Read the model definition and answer for the solid it produces. Units are mm, in the model's axes. Coordinates: 2 decimals unless noted, no trailing zeros. Loops run counter-clockwise (first coordinate to the right, second up) from the corner with the lowest first, then second, coordinate; pieces in that order, holes last.
Q1. Section B-B (y = 22.5) is taken. Give the vertices of the cut face in (x, z).
Q2. Flat-ended cylindrical pins translate along their axes: P1, Ø1.5, axis at x = 2, z = -83, coming from the -Y side; P2, Ø1.5, axis at x = 1.5, z = -104.5, coming from the -Y side. Find the tip coordinate at first contact, or state that the pin passes through.
Q3. Straight lines are drawn through the part: line 1 (Z direction, x = 0.4, y = 9); line 2 (Y direction, x = 2.55, z = -91). For each, find the intervals that lie inside material, in ascending order.
Q4. Section A-A (x = 0.5) is taken. Give the vertices of the cut face in (y, z).
Autodesk Inventor part; units mm, degrees
ref_plane "YZ Plane" through (0, 0, 0) normal (1, 0, 0) x (0, 1, 0)
ref_plane "XZ Plane" through (0, 0, 0) normal (0, 1, 0) x (-1, 0, 0)
ref_plane "XY Plane" through (0, 0, 0) normal (0, 0, 1) x (1, 0, 0)
sketch "Boceto1" plane through (0, 0, 0) normal (1, 0, 0) x (0, 1, 0)
  line L0 (0, 0) -> (24.8, 0)
  line L1 (24.8, 0) -> (24.8, -89.7)
  line L2 (24.8, -89.7) -> (0, -89.7)
  line L3 (0, -89.7) -> (0, 0)
  line L4 (0, -44.85) -> (73, -44.85) construction
  line L5 (24.8, -44.85) -> (73, -44.85) construction
  line L6 (24.8, 25.15) -> (73, 25.15)
  line L7 (73, 25.15) -> (73, -114.85)
  line L8 (73, -114.85) -> (24.8, -114.85)
  line L9 (24.8, -114.85) -> (24.8, 25.15)
  line L10 (24.8, 25.15) -> (73, -114.85) construction
  line L11 (73, 25.15) -> (24.8, -114.85) construction
  point P0 (48.9, -44.85)
  dimension "d0" = 24.8
  dimension "d1" = 89.7
  dimension "d2" = 73
  dimension "d3" = 140
extrude "Extrusión1" add sketch "Boceto1" along normal blind 3
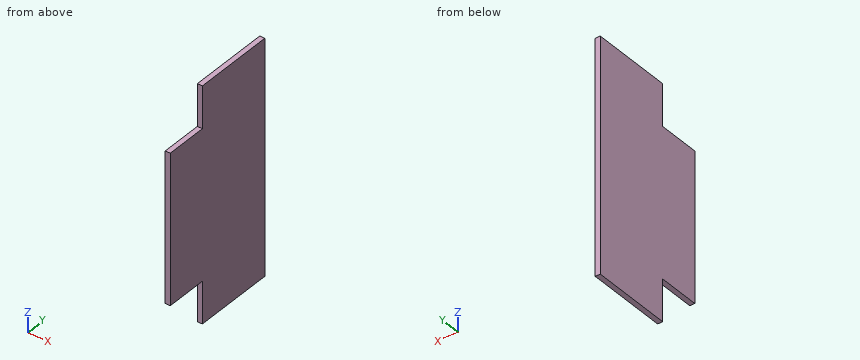
Numbers:
1. outline: (0, -89.7) - (3, -89.7) - (3, 0) - (0, 0) - close
2. P1: stops at y = 0
2. P2: stops at y = 24.8
3. line 1: z = -89.7 to 0
3. line 2: y = 24.8 to 73
4. outline: (0, -89.7) - (24.8, -89.7) - (24.8, -114.85) - (73, -114.85) - (73, 25.15) - (24.8, 25.15) - (24.8, 0) - (0, 0) - close
